The drawing under review shows one solid part. Ordinate dimensions are in mm from its lowest x, y, z. Coordinates: 2 decimals unless noted, no trailing zeros. Write each loop counter-clockwise with the first axis right and the second up, starting at its lowest first coordinate (ties: lowest second). Pieces come first, ordered by that corner, then holes.
Q1. Add section C-C, the plane y = 1.1. Give the boundary of the cut face in (x, z) (1 decimal), plus the area to 3 significant figures.
Q2. Add section D-D, the plane z = 26.5. Give the boundary of the cut face in (x, y), plus the area to 3 significant figures.
Q3. Add section B-B, the plane z = 6.5. Give the boundary of the cut face in (x, y) (1 decimal).
Q4. Clearance check with a flat-ended pin moving along its axis: pin 1 Ø1 at (x, y) = (22.5, 1) entering from -Z. State where the tip first meets the part, or that it passes through.
Q5. Add section A-A, the plane x = 39. Give the boundary of the cut face in (y, z).
Q6. To check wall thickness, follow probe 1 along X at (y, z) = (1.4, 21) (1 decimal); probe 2 along X at (y, z) = (1.7, 18); probe 3 along Z at (x, y) = (19, 2.25) (1 decimal). State the ranges of each line that lie inside material, in increasing order.
Q7. The part is to be moulded in two halves that separate along X. For the marked faces 1, 2 and 3, say which applies: +X half, -X half, draft (parallel to the pull), parting line (faces both ways), or undercut.
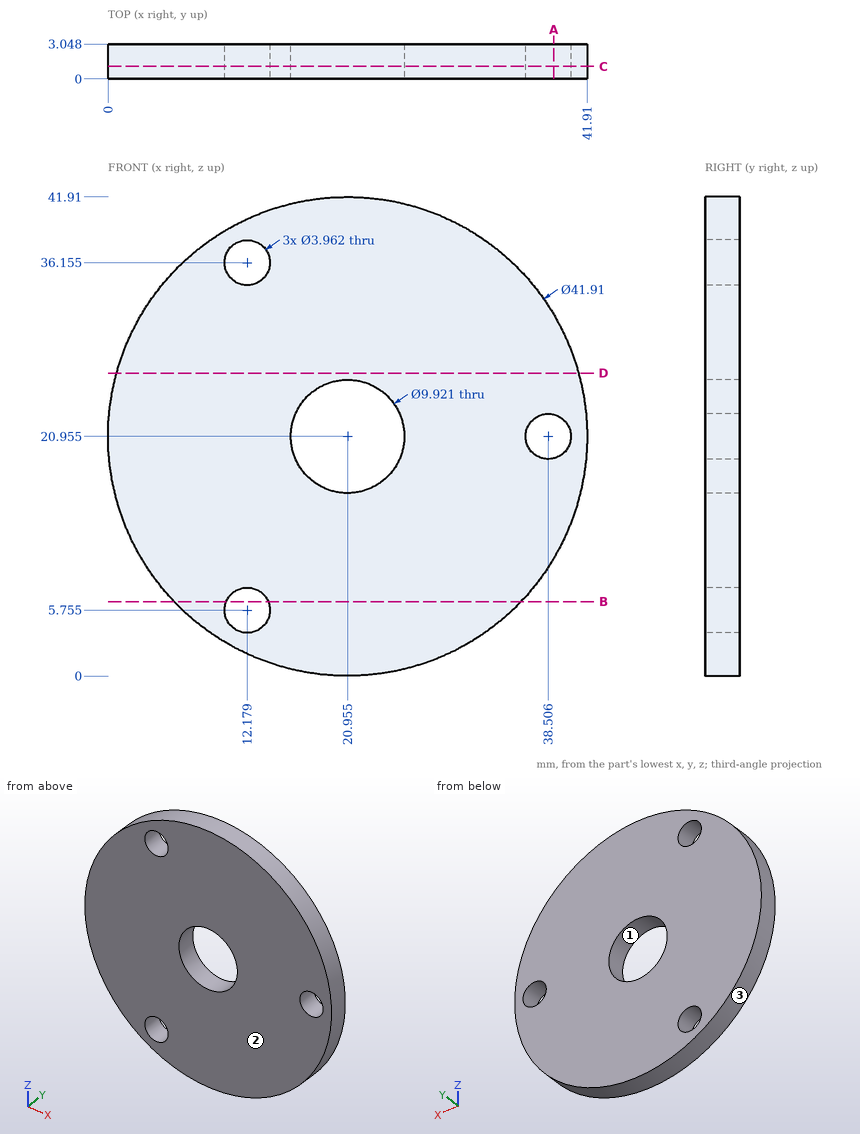
Here are the results:
1. outline: circle Ø41.9 at (21, 21); hole circle Ø4 at (12.2, 5.8); hole circle Ø4 at (12.2, 36.2); hole circle Ø9.9 at (21, 21); hole circle Ø4 at (38.5, 21)
1. area: 1,270 mm2
2. outline: (0.75, 0) - (41.16, 0) - (41.16, 3.05) - (0.75, 3.05) - close
2. area: 123 mm2
3. outline: (5.8, 0) - (10.3, 0) - (10.3, 3) - (5.8, 3) - close; (14, 0) - (36.1, 0) - (36.1, 3) - (14, 3) - close
4. pin 1: stops at z = 0.03
5. outline: (0, 10.3) - (3.05, 10.3) - (3.05, 19.04) - (0, 19.04) - close; (0, 22.87) - (3.05, 22.87) - (3.05, 31.61) - (0, 31.61) - close
6. probe 1: x = 0 to 16, 25.9 to 36.5, 40.5 to 41.9
6. probe 2: x = 0.21 to 16.97, 24.94 to 41.7
6. probe 3: z = 0.1 to 16.4, 25.5 to 41.8
7. face 1: undercut
7. face 2: draft
7. face 3: parting line
